```python
from build123d import *

# Parameters (mm, degrees)
F0_R     = 9.525
F1_DEPTH = 12.7
F2_R     = 8.255
F3_DEPTH = 10.16
F4_R     = 5.55625
F5_DEPTH = 25.4
F7_R     = 1.524
F8_DEPTH = 10.16


with BuildPart() as f1:
    # F0 (on Top) → F1 (new body)
    with BuildSketch(Plane.XY):
        Circle(F0_R)
    extrude(amount=F1_DEPTH)

    # F2 (on face) → F3 (cut)
    with BuildSketch(Plane.XY.offset(12.7)):
        Circle(F2_R)
    extrude(amount=-F3_DEPTH, mode=Mode.SUBTRACT)

    # F4 (on face) → F5 (cut)
    with BuildSketch(Plane.XY.offset(2.54)):
        Circle(F4_R)
    extrude(amount=-F5_DEPTH, mode=Mode.SUBTRACT)

    # F7 (on offset) → F8 (join)
    with BuildSketch(Plane.YZ.offset(9.271)):
        with Locations((0, 5.842)):
            Circle(F7_R)
    extrude(amount=F8_DEPTH)

    # F9: F1 across plane


with BuildPart() as f1_1:
    add(f1.part)
    add(f1.part.mirror(Plane.YZ))


solid = f1_1.part
```
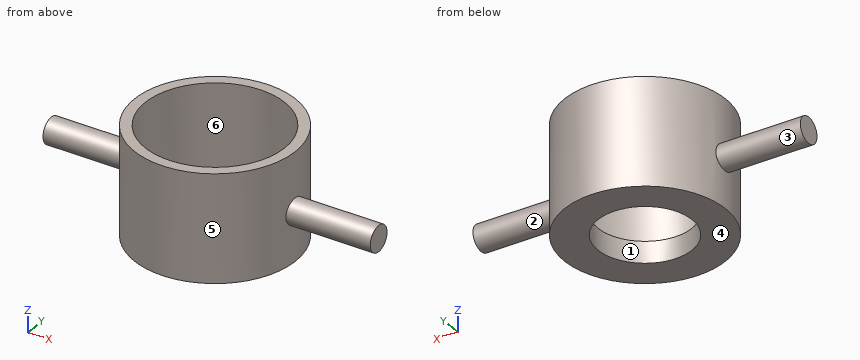
Read the model definition and answer for the solid it produces. Units are mm, in the model's axes. Face numbers are marked on the shaded views. A direction names the side the tool comes from. Coordinates: 2 decimals unless noted, no trailing zeros. Loops run counter-clockwise (first coordinate to the right, second up) from the corner with the lowest first, then second, coordinate; pieces in that order, holes last.
(1) Flat-ended cylindrical pins translate along their axes: pin 1 Ø8 at (x, y) = (-1, -2.5) entering from +Z; pin 2 Ø1 at (x, y) = (-11, 3) entering from +Z; pin 3 Ø4 at (x, z) = (-9.5, 1.5) entering from -Y; pin 4 Ø4 at (y, z) = (-6.5, 10.5) entering from +X (3 decimals). Find the tip coordinate at first contact, or state that the pin passes through.
Solution:
pin 1: stops at z = 2.54
pin 2: passes through
pin 3: stops at y = -5.87
pin 4: stops at x = 8.395
(2) Consider line 1 along Y through (x, z) = (0, 7.5) (3 decimals); line 2 along Y through (x, z) = (0, 1.65) (3 decimals); line 3 along X through (y, z) = (0, 6.5) (3 decimals). Determine where each line is inside the solid, lowest interval first.
Solution:
line 1: y = -9.525 to -8.255, 8.255 to 9.525
line 2: y = -9.525 to -5.556, 5.556 to 9.525
line 3: x = -19.431 to -8.255, 8.255 to 19.431
(3) The mould has two halves that part along X. Classify the marked faces 4, 5 and 6: released by +X, released by -X, zero draft, split by the parting line, or undercut.
Solution:
face 4: zero draft
face 5: split by the parting line
face 6: undercut
(4) The part is cut by section D-D (x = -6.5). Determine the outline of the cut face in (y, z).
Solution:
outline: (-6.96, 0) - (6.96, 0) - (6.96, 12.7) - (5.09, 12.7) - (5.09, 2.54) - (-5.09, 2.54) - (-5.09, 12.7) - (-6.96, 12.7) - close
(5) The part is cut by section B-B (x = 0). Determine the outline of the cut face in (y, z) (3 decimals), and give its area (3 significant figures).
Solution:
outline: (-9.525, 0) - (-5.556, 0) - (-5.556, 2.54) - (-8.255, 2.54) - (-8.255, 12.7) - (-9.525, 12.7) - close; (5.556, 0) - (9.525, 0) - (9.525, 12.7) - (8.255, 12.7) - (8.255, 2.54) - (5.556, 2.54) - close
area: 46.0 mm2
(6) The part is cut by section A-A (y = 0). Determine the outline of the cut face in (x, z) (3 decimals), and give its area (3 significant figures).
Solution:
outline: (-19.431, 4.318) - (-9.525, 4.318) - (-9.525, 0) - (-5.556, 0) - (-5.556, 2.54) - (-8.255, 2.54) - (-8.255, 12.7) - (-9.525, 12.7) - (-9.525, 7.366) - (-19.431, 7.366) - close; (5.556, 0) - (9.525, 0) - (9.525, 4.318) - (19.431, 4.318) - (19.431, 7.366) - (9.525, 7.366) - (9.525, 12.7) - (8.255, 12.7) - (8.255, 2.54) - (5.556, 2.54) - close
area: 106 mm2
(7) The part is cut by section C-C (z = 9.5). Determine the outline of the cut face in (x, y) (3 decimals), and give its area (3 significant figures).
Solution:
outline: circle Ø19.05 at (0, 0); hole circle Ø16.51 at (0, 0)
area: 70.9 mm2
(8) A tool of negligible diameter and unlimited length cuts with its end or side. For the marked faces 1, 2 and 3, from which of +Z, -Z, +X, -X, +Y, -Y can it reach the whole face along a straight path? Write none if from no direction.
Solution:
face 1: +Z, -Z
face 2: +X
face 3: -X
